```python
from build123d import *

# Parameters (mm, degrees)
SKETCH1_W           = 35
SKETCH1_H           = 20
SKETCH1_R           = 1.5
BOSS_EXTRUDE1_DEPTH = 1.57
SKETCH2_R           = 10
BOSS_EXTRUDE2_DEPTH = 15.34
SKETCH3_W           = 3
SKETCH3_H           = 9.75
BOSS_EXTRUDE3_DEPTH = 4.6
SKETCH4_W           = 8.75
SKETCH4_H           = 3.6
BOSS_EXTRUDE4_DEPTH = 4.82
SKETCH5_W           = 1.666666667
SKETCH5_H           = 3.6
SKETCH5_W_2         = 1.666666666
SKETCH5_W_3         = 1.416666667
CUT_EXTRUDE1_DEPTH  = 4.82
SKETCH6_R           = 1.29689407
SKETCH6_R_2         = 1.720847255
SKETCH6_R_3         = 1.291006222
SKETCH6_R_4         = 1.284790683
BOSS_EXTRUDE5_DEPTH = 6
SKETCH7_R           = 2.5
BOSS_EXTRUDE6_DEPTH = 2


with BuildPart() as part:
    # Sketch1 → Boss-Extrude1 (new body)
    with BuildSketch(Plane(origin=(0, 0, 0), x_dir=(1, 0, 0), z_dir=(0, 1, 0))):
        with Locations((17.5, 10)):
            Rectangle(SKETCH1_W, SKETCH1_H)
        with Locations(Location((2.3, 17.7, 0), (0, 0, 270))):
            Circle(SKETCH1_R, mode=Mode.SUBTRACT)
        with Locations(Location((2.3, 2.3, 0), (0, 0, 270))):
            Circle(SKETCH1_R, mode=Mode.SUBTRACT)
    extrude(amount=BOSS_EXTRUDE1_DEPTH)

    # Sketch2 → Boss-Extrude2 (add)
    with BuildSketch(Plane(origin=(0, 1.57, 0), x_dir=(1, 0, 0), z_dir=(0, 1, 0))):
        with Locations(Location((25, 10, 0), (0, 0, 270))):
            Circle(SKETCH2_R)
    extrude(amount=BOSS_EXTRUDE2_DEPTH)

    # Sketch3 → Boss-Extrude3 (add)
    with BuildSketch(Plane(origin=(0, 1.57, 0), x_dir=(1, 0, 0), z_dir=(0, 1, 0))):
        with Locations((2.5, 10)):
            Rectangle(SKETCH3_W, SKETCH3_H)
    extrude(amount=BOSS_EXTRUDE3_DEPTH)

    # Sketch4 → Boss-Extrude4 (add)
    with BuildSketch(Plane.ZY.offset(-1)):
        with Locations((-10, 3.87)):
            Rectangle(SKETCH4_W, SKETCH4_H)
    extrude(amount=BOSS_EXTRUDE4_DEPTH)

    # Sketch5 → Cut-Extrude1 (cut)
    with BuildSketch(Plane.ZY.offset(3.82)):
        with Locations((-12.541666666, 3.87)):
            Rectangle(SKETCH5_W, SKETCH5_H)
        with Locations((-9.875, 3.87)):
            Rectangle(SKETCH5_W_2, SKETCH5_H)
        with Locations((-7.333333334, 3.87)):
            Rectangle(SKETCH5_W_3, SKETCH5_H)
    extrude(amount=-CUT_EXTRUDE1_DEPTH, mode=Mode.SUBTRACT)

    # Sketch6 → Boss-Extrude5 (add)
    with BuildSketch(Plane(origin=(0, 1.57, 0), x_dir=(1, 0, 0), z_dir=(0, 1, 0))):
        with Locations(Location((12.406689858, 7.897918268, 0), (0, 0, 90))):
            Circle(SKETCH6_R)
        with Locations(Location((11.577372326, 12.210536894, 0), (0, 0, 90))):
            Circle(SKETCH6_R_2)
        with Locations(Location((10.375255256, 5.440145452, 0), (0, 0, 90))):
            Circle(SKETCH6_R_3)
        with Locations(Location((9.342761815, 8.766255662, 0), (0, 0, 90))):
            Circle(SKETCH6_R_4)
    extrude(amount=BOSS_EXTRUDE5_DEPTH)

    # Sketch7 → Boss-Extrude6 (add)
    with BuildSketch(Plane.XZ):
        with Locations(Location((25, -10, 0), (0, 0, 270))):
            Circle(SKETCH7_R)
    extrude(amount=BOSS_EXTRUDE6_DEPTH)


solid = part.part
```
Check sheet for the modelled part. Datum: model origin and axes. Units: mm. A direction names the side the tool comes from. Give positions to 0.01 mm unless a question says otherwise; leave off trailing zeros. Write each loop counter-clockwise with the first axis right and the second up, starting at its lowest first coordinate (ties: lowest second). Pieces come first, ordered by that corner, then holes. Notation, with made-up numbers: (80.25, 73.25) - (135.25, 73.25) arc R23 cw to (135.25, 112.25) - close; hole circle Ø4 at (-32, 7). An arc over 180 degrees is marked (long way). Answer as a JSON object with one key per item and string values. Group by question number.
1) Access from +Z, -Z, +X, -X, +Y, -Y to the whole of each face (thin tool, end or side, straight path). Record for faces 4 (the face through (-1, 4, -14.375)), 5 (the face through (10, 7.57, -5)), 6 (the face through (4, 4, -10)), 7 (the face through (2, 4, -5.125)), 8 (the face through (-1, 4, -11.708)).
2) Thickness scan on probe 1 along X at (y, z) = (0.8, -2.3); probe 2 along Y at (x, z) = (25, -19); probe 3 along Y at (x, z) = (2, -5.25). Record the ranges inside material, lowest first. Write a range as from..to.
3) Sectioned sample at B-B (z = -2.3). Record the cut outline in (x, y).
4) Sectioned sample at D-D (y = -0.5). Record the cut outline in (x, z).
5) Sectioned sample at C-C (y = 5.25). Record the cut outline in (x, z) (3 decimals).
6) Depth check by flat-ended pin: P1, Ø1.8, axis at x = -2, y = 3, coming from the -Z side (3 decimals); P2, Ø6, axis at y = 6, z = -12, coming from the -X side; P3, Ø3, axis at x = -1, y = 4, coming from the +Z side (3 decimals); P4, Ø1, axis at x = 2.5, y = 7, coming from the +Z side. Enter the tip coordinate at first touch or a pass-through.
7) Sectioned sample at A-A (x = 2.3). Record the cut outline in (y, z) (3 decimals), then the cut area to 3 significant figures.
8) Release check for a two-part mould opening along X. For faces 1 (the face through (12, 7.57, -8)), 2 (the face through (-3.82, 4, -11)), 3 (the face through (9.287, 4.528, -6.134)) record: pulls with the +X half, pulls with the -X half, needs draft (parallel to the pull), parting line crosses it, or undercut.
Geometry results:
{
 "1": {"face 4": "-Z, -X, +Y", "face 5": "+Z, -Z, -X, +Y", "face 6": "+Z, -Z, +Y", "face 7": "+Z, -X, +Y", "face 8": "-X, +Y"},
 "2": {"probe 1": "x = 0..0.8, 3.8..35", "probe 2": "y = 0..16.91", "probe 3": "y = 0..6.17"},
 "3": {"outline": "(0, 0) - (0.8, 0) - (0.8, 1.57) - (0, 1.57) - close; (3.8, 0) - (35, 0) - (35, 1.57) - (31.38, 1.57) - (31.38, 16.91) - (18.62, 16.91) - (18.62, 1.57) - (3.8, 1.57) - close"},
 "4": {"outline": "circle Ø5 at (25, -10)"},
 "5": {"outline": "(-3.82, -14.375) - (1, -14.375) - (1, -14.875) - (4, -14.875) - (4, -5.125) - (1, -5.125) - (1, -5.625) - (-3.82, -5.625) - (-3.82, -6.625) - (1, -6.625) - (1, -8.042) - (-3.82, -8.042) - (-3.82, -9.042) - (1, -9.042) - (1, -10.708) - (-3.82, -10.708) - (-3.82, -11.708) - (1, -11.708) - (1, -13.375) - (-3.82, -13.375) - close; circle Ø2.57 at (9.343, -8.766); circle Ø2.582 at (10.375, -5.44); circle Ø3.442 at (11.577, -12.211); circle Ø2.594 at (12.407, -7.898); circle Ø20 at (25, -10)"},
 "6": {"P1": "stops at z = -14.375", "P2": "stops at x = -3.82", "P3": "stops at z = -5.625", "P4": "passes through"},
 "7": {"outline": "(0, -20) - (1.57, -20) - (1.57, -19.2) - (0, -19.2) - close; (0, -16.2) - (1.57, -16.2) - (1.57, -14.875) - (6.17, -14.875) - (6.17, -5.125) - (1.57, -5.125) - (1.57, -3.8) - (0, -3.8) - close; (0, -0.8) - (1.57, -0.8) - (1.57, 0) - (0, 0) - close", "area": "66.8 mm^2"},
 "8": {"face 1": "needs draft", "face 2": "pulls with the -X half", "face 3": "undercut"}
}
